Here's the drawing with two shaded views (mm, measured from the low corner). I have some questions. A direction names the side the tool comes from. Round coordinates to 2 decimals unless told otherwise and drop trailing zeros. Loops run counter-clockwise (first coordinate to the right, second up) from the corner with the lowest first, then second, coordinate; pieces in that order, holes last. Notation, with made-up numbers: M -32,-20.5 L -7,-20.5 A19 cw -7,-1.5 Z; hole C 78.25,75 d7. An arc over 180 degrees is marked long. Answer as a JSON object with one key per item and string values.
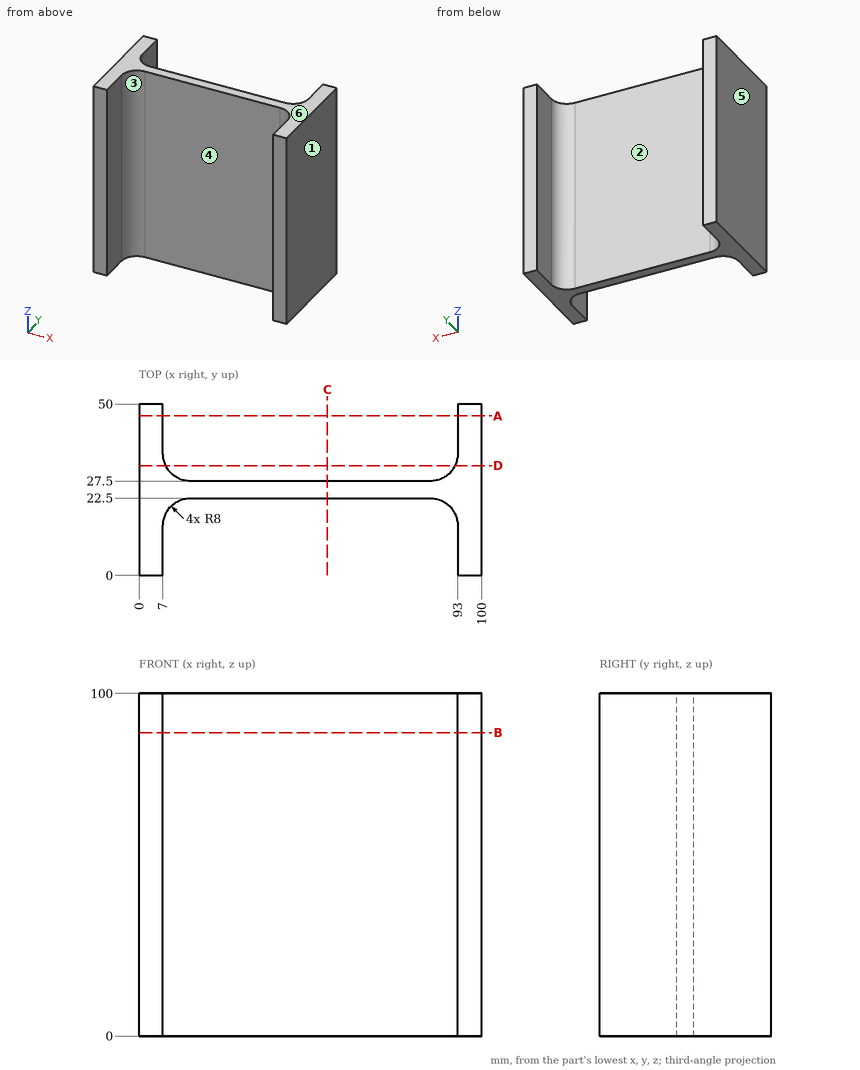
Item 1: We'd pull the mould along X, two halves only. Please class the marked faces 4, 5 and 6: +X half, -X half, draft (parallel to the pull), parting line (faces both ways), or undercut.
Solution:
{"face 4": "undercut", "face 5": "-X half", "face 6": "draft"}
Item 2: For P1, Ø16, axis at y = 9, z = 67.5, coming from the -X side; P2, Ø6, axis at x = 63.5, z = 27, coming from the -Y side; P3, Ø6, axis at x = 56, z = 87.5, coming from the +Y side, each with a flat end and sliding along its axis, tell me the tip position at first contact or that it passes through.
Solution:
{"P1": "stops at x = 0", "P2": "stops at y = 22.5", "P3": "stops at y = 27.5"}
Item 3: I want a section at A-A on y = 46.5. List the corners of the cut face in (x, z) for me.
Solution:
{"outline": "M 0,0 L 7,0 L 7,100 L 0,100 Z; M 93,0 L 100,0 L 100,100 L 93,100 Z"}
Item 4: I want a section at C-C on x = 55. List the corners of the cut face in (y, z) for me, plus the area to 3 significant figures.
Solution:
{"outline": "M 22.5,0 L 27.5,0 L 27.5,100 L 22.5,100 Z", "area": "500 mm2"}
Item 5: I want a section at B-B on z = 88.5. List the corners of the cut face in (x, y) for me.
Solution:
{"outline": "M 0,0 L 7,0 L 7,14.5 A8 cw 15,22.5 L 85,22.5 A8 cw 93,14.5 L 93,0 L 100,0 L 100,50 L 93,50 L 93,35.5 A8 cw 85,27.5 L 15,27.5 A8 cw 7,35.5 L 7,50 L 0,50 Z"}
Item 6: If I drill on L1, parallel to X at y = 9, z = 58.5; L2, parallel to Y at x = 63, z = 89; L3, parallel to X at y = 32.5, z = 49, over which ranges is the centre line in solid material (lowest first)? Write a range as from..to.
Solution:
{"L1": "x = 0..7, 93..100", "L2": "y = 22.5..27.5", "L3": "x = 0..7.58, 92.42..100"}
Item 7: For the marked faces 1, 2 and 3, which set-ups out of +Z, -Z, +X, -X, +Y, -Y let a thin tool reach every point of the face, with its end or its side?
Solution:
{"face 1": "+Z, -Z, +X, +Y, -Y", "face 2": "+Z, -Z, +Y", "face 3": "+Z, -Z, -Y"}
Item 8: I want a section at D-D on y = 32. List the corners of the cut face in (x, z) for me.
Solution:
{"outline": "M 0,0 L 7.81,0 L 7.81,100 L 0,100 Z; M 92.19,0 L 100,0 L 100,100 L 92.19,100 Z"}
